Check sheet for the modelled part. Datum: model origin and axes. Units: mm. A direction names the side the tool comes from. Coordinates: 2 decimals unless noted, no trailing zeros. Write each loop counter-clockwise with the first axis right and the second up, starting at its lowest first coordinate (ties: lowest second). Pieces come first, ordered by that corner, then holes. Notation, with made-up numbers: M -37.5,64 L -11.5,64 A15 ccw -11.5,79 Z; hole C 81,-19.75 d3. An arc over 180 degrees is marked long. Answer as CSV lines item,"result". Start each with the question number.
1) Section check B-B (y = -3.75). Record the cut outline in (x, z), and give its area (3 significant figures).
2) Section check C-C (x = -2.5). Record the cut outline in (y, z), and give its area (3 significant figures).
3) Material ranges on L1, parallel to Y at x = -22.5, z = 2.25; L2, parallel to Y at x = -26.5, z = 3; L3, parallel to X at y = -3, z = 0.5, recorded low to high. Write a range as [from, to].
4) Go/stop test with flat-tipped pins: pin 1 Ø3 at (x, z) = (33.5, 2.5) entering from +Y; pin 2 Ø3 at (x, z) = (14.5, 2.5) entering from -Y; pin 3 Ø3 at (y, z) = (-9, 4) entering from -X. Record where each tip stops, or that it passes through.
5) Section check A-A (y = 9). State how many separate pieces and enclosed holes the cut face has, and give its area (3 significant figures).
6) Access from +Z, -Z, +X, -X, +Y, -Y to the whole of each face (thin tool, end or side, straight path). Record for faces 1 (the flat face through (63.5, 9, 3)), 2 (the flat face through (67, -6.35, 3)), 3 (the flat face through (31.75, -10, 3)).
from build123d import *

# Parameters (mm, degrees)
BOSS_EXTRUDE1_DEPTH = 6.35


with BuildPart() as part:
    # Sketch1 → Boss-Extrude1 (new body)
    with BuildSketch(Plane.XY):
        Polygon((-76.2, 12.7), (-63.5, 12.7), (-63.5, 6.35), (-57.15, 6.35), (-57.15, 12.7), (-50.8, 12.7), (-50.8, 6.35), (-44.45, 6.35), (-44.45, 12.7), (-38.1, 12.7), (-38.1, 6.35), (-31.75, 6.35), (-31.75, 12.7), (-25.4, 12.7), (-25.4, 6.35), (-19.05, 6.35), (-19.05, 12.7), (-12.7, 12.7), (-12.7, 6.35), (-6.35, 6.35), (-6.35, 12.7), (6.35, 12.7), (6.35, 6.35), (12.7, 6.35), (12.7, 12.7), (19.05, 12.7), (19.05, 6.35), (25.4, 6.35), (25.4, 12.7), (31.75, 12.7), (31.75, 6.35), (38.1, 6.35), (38.1, 12.7), (44.45, 12.7), (44.45, 6.35), (50.8, 6.35), (50.8, 12.7), (57.15, 12.7), (57.15, 6.35), (63.5, 6.35), (63.5, 12.7), (76.2, 12.7), (76.2, 0), (69.85, 0), (69.85, -6.35), (63.5, -6.35), (63.5, -12.7), (57.15, -12.7), (57.15, -6.35), (50.8, -6.35), (50.8, -12.7), (44.45, -12.7), (44.45, -6.35), (38.1, -6.35), (38.1, -12.7), (31.75, -12.7), (31.75, -6.35), (25.4, -6.35), (25.4, -12.7), (19.05, -12.7), (19.05, -6.35), (12.7, -6.35), (12.7, -12.7), (6.35, -12.7), (6.35, -6.35), (-6.35, -6.35), (-6.35, -12.7), (-12.7, -12.7), (-12.7, -6.35), (-19.05, -6.35), (-19.05, -12.7), (-25.4, -12.7), (-25.4, -6.35), (-31.75, -6.35), (-31.75, -12.7), (-38.1, -12.7), (-38.1, -6.35), (-44.45, -6.35), (-44.45, -12.7), (-50.8, -12.7), (-50.8, -6.35), (-57.15, -6.35), (-57.15, -12.7), (-63.5, -12.7), (-63.5, -6.35), (-69.85, -6.35), (-69.85, 0), (-76.2, 0), align=None)
    extrude(amount=BOSS_EXTRUDE1_DEPTH)


solid = part.part
Results found:
1,outline,"M -69.85,0 L 69.85,0 L 69.85,6.35 L -69.85,6.35 Z"
1,area,"887 mm2"
2,outline,"M -6.35,0 L 12.7,0 L 12.7,6.35 L -6.35,6.35 Z"
2,area,"121 mm2"
3,L1,"y = [-12.7, 6.35]"
3,L2,"y = [-6.35, 12.7]"
3,L3,"x = [-69.85, 69.85]"
4,pin 1,"stops at y = 6.35"
4,pin 2,"stops at y = -6.35"
4,pin 3,"stops at x = -63.5"
5,separate pieces,"11"
5,enclosed holes,"0"
5,area,"565 mm2"
6,face 1,"+Z, -Z, +Y"
6,face 2,"+Z, -Z, +X, -Y"
6,face 3,"+Z, -Z, -Y"
